Design review of the part shown in the three views and the two pictorial views. Dimensions are in mm from the part's minimum x, y and z. A direction names the side the tool comes from. Give positions to 0.01 mm unless a question says otherwise; leave off trailing zeros. Order: outer loops, then holes, each group sorted by start corner. A loop starts at its lowest first (then second) coordinate and runs counter-clockwise, first axis right, second up.
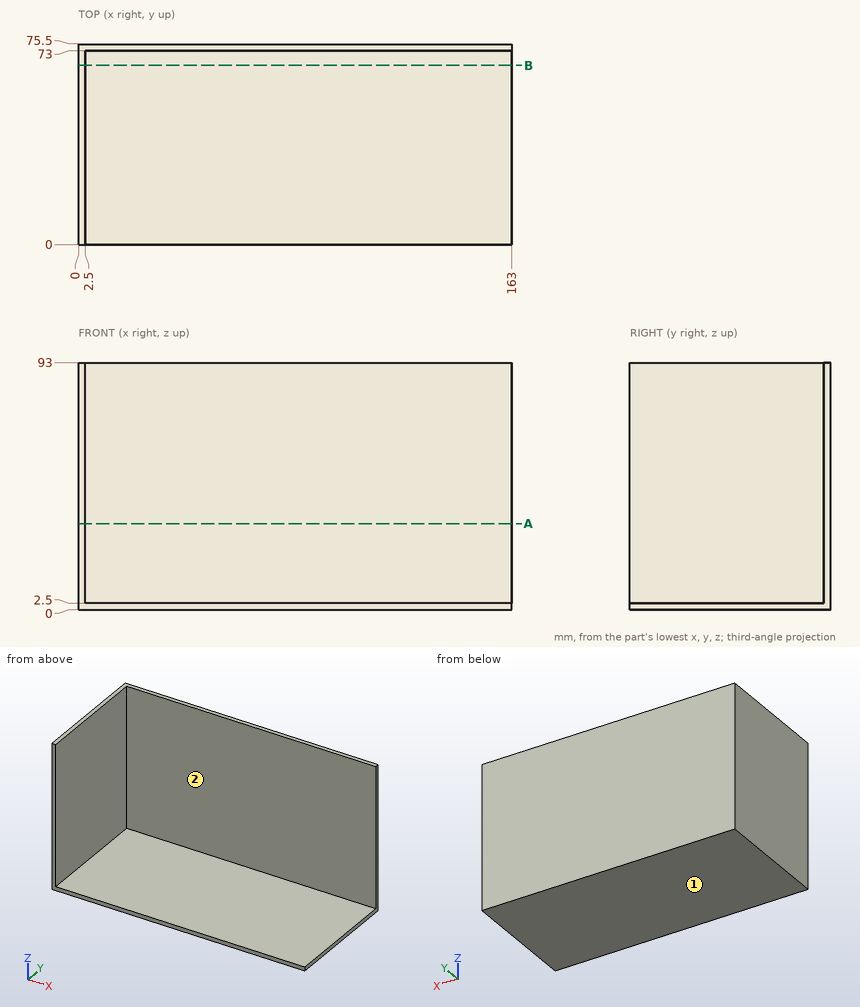
1) We need section A-A on z = 32.5. Give the boundary of the cut face in (x, y).
Answer sheet:
outline: (0, 0) - (2.5, 0) - (2.5, 73) - (163, 73) - (163, 75.5) - (0, 75.5) - close
2) Clearance check with flat-ended pins moving along their axes: pin 1 (8 mm diameter, centred on x = 51.5, z = 22, fed in from -Y); pin 2 (12 mm diameter, centred on x = 61.5, y = 10.5, fed in from +Z); pin 3 (3 mm diameter, centred on y = 50.5, z = 75, fed in from +X). State where each tip first meets the part, or that it passes through.
Answer sheet:
pin 1: stops at y = 73
pin 2: stops at z = 2.5
pin 3: stops at x = 2.5
3) To check wall thickness, follow line 1 (Z direction, x = 101, y = 21); line 2 (Y direction, x = 97, z = 62.5). State the ranges of each line that lie inside material, in increasing order.
Answer sheet:
line 1: z = 0 to 2.5
line 2: y = 73 to 75.5
4) We need section B-B on y = 67.5. Give the boundary of the cut face in (x, z), then the cut area to 3 significant figures.
Answer sheet:
outline: (0, 0) - (163, 0) - (163, 2.5) - (2.5, 2.5) - (2.5, 93) - (0, 93) - close
area: 634 mm2
5) Tool access review of the marked faces 1 and 2: name each direction out of +Z, -Z, +X, -X, +Y, -Y from which nothing blocks a thin tool from reaching the whole face with its end or side.
Answer sheet:
face 1: -Z, +X, -X, +Y, -Y
face 2: +Z, +X, -Y
